Part model, mm, in its own coordinate system. A direction names the side the tool comes from. Coordinates: 2 decimals unless noted, no trailing zeros. Loops run counter-clockwise (first coordinate to the right, second up) from the corner with the lowest first, then second, coordinate; pieces in that order, holes last. Notation, with made-up numbers: (63, -18) -> (67, -18) arc R32 cw to (67, 19) -> close; hole circle Ø6 at (-16, 37). An arc over 180 degrees is marked (long way). Use one line per item in the form item = value. Start each with the question number.
(1) 3-axis set-ups, long thin cutter, end or side, ignore diameter. For faces 1 (the flat face through (50.8, 13, 2)), 2 (the cylindrical face through (40.561, 37.325, 1.565)): which of +Z, -Z, +X, -X, +Y, -Y reach the whole face in a straight line?
(2) Band-saw the part on C-C on y = 19. Give the cut face in (x, z) (3 decimals).
(3) Drill centre lines: L1, parallel to Y at x = 12.7, z = 1.55; L2, parallel to X at y = 17.5, z = 2.65; L3, parallel to Y at x = 30, z = 1.85. Where is each one in solid material? Low to high. Write a range as [from, to].
(4) Band-saw the part on B-B on x = 12.7. Give the cut face in (y, z) (3 decimals), then the cut area to 3 significant figures.
(5) Mould opens along X. For faces 3 (the cylindrical face through (62, 36, 2)), 4 (the flat face through (13, 0, 2)), 5 (the flat face through (76.2, 25, 2)) say: +X half, -X half, draft (parallel to the pull), parting line (faces both ways), or undercut.
(6) Pin check, flat tips, straight feed: P1, Ø4.5, axis at x = 63.5, y = 38.1, coming from the -Z side; P2, Ø1, axis at x = 34, z = 1, coming from the -Y side. Stop position of each tip, or through.
(7) Band-saw the part on A-A on y = 12.7. Give the cut face in (x, z) (3 decimals).
(8) Band-saw the part on D-D on z = 1.35. Give the cut face in (x, y), then the cut area to 3 significant figures.
Autodesk Inventor part; units mm, degrees
ref_plane "YZ Plane" through (0, 0, 0) normal (1, 0, 0) x (0, 1, 0)
ref_plane "XZ Plane" through (0, 0, 0) normal (0, 1, 0) x (-1, 0, 0)
ref_plane "XY Plane" through (0, 0, 0) normal (0, 0, 1) x (1, 0, 0)
sketch "Sketch1" plane through (0, 0, 0) normal (0, 0, 1) x (1, 0, 0)
  line L0 (0, 0) -> (25.4, 0)
  line L1 (25.4, 0) -> (25.4, 25.4)
  line L2 (25.4, 50.8) -> (0, 50.8)
  line L3 (0, 50.8) -> (0, 0)
  line L4 (0, 25.4) -> (0, 50.8)
  line L5 (12.7, 0) -> (12.7, 12.7) construction
  line L6 (12.7, 12.7) -> (12.7, 38.1) construction
  line L7 (12.7, 38.1) -> (38.1, 38.1) construction
  circle A0 centre (12.7, 12.7) radius 2.5797
  circle A1 centre (12.7, 38.1) radius 2.5797
  circle A2 centre (38.1, 38.1) radius 2.5797
  line L8 (25.4, 25.4) -> (50.8, 25.4)
  line L9 (50.8, 25.4) -> (50.8, 0)
  line L10 (50.8, 0) -> (76.2, 0)
  line L11 (76.2, 0) -> (76.2, 50.8)
  line L12 (76.2, 50.8) -> (25.4, 50.8)
  line L13 (38.1, 38.1) -> (63.5, 38.1) construction
  line L14 (63.5, 38.1) -> (63.5, 12.7) construction
  circle A3 centre (63.5, 38.1) radius 2.5797
  circle A4 centre (63.5, 12.7) radius 2.5797
  dimension "d0" = 25.4
  dimension "d1" = 50.8
  dimension "d5" = 12.7
  dimension "d6" = 25.4
  dimension "d7" = 25.4
  dimension "d11" = 5.1594
  dimension "d14" = 25.4
  dimension "d15" = 25.4
  dimension "d16" = 25.4
  dimension "d17" = 25.4
extrude "Extrusion2" add sketch "Sketch1" along normal blind 3.175
properties part number "C-Bracket"
A:
q1.face_1 = +Z, -Z, -Y
q1.face_2 = +Z, -Z
q2.outline = (0, 0) -> (25.4, 0) -> (25.4, 3.175) -> (0, 3.175) -> close; (50.8, 0) -> (76.2, 0) -> (76.2, 3.175) -> (50.8, 3.175) -> close
q3.L1 = [0, 10.12], [15.28, 35.52], [40.68, 50.8]
q3.L2 = [0, 25.4], [50.8, 76.2]
q3.L3 = [25.4, 50.8]
q4.outline = (0, 0) -> (10.12, 0) -> (10.12, 3.175) -> (0, 3.175) -> close; (15.28, 0) -> (35.52, 0) -> (35.52, 3.175) -> (15.28, 3.175) -> close; (40.68, 0) -> (50.8, 0) -> (50.8, 3.175) -> (40.68, 3.175) -> close
q4.area = 129 mm²
q5.face_3 = undercut
q5.face_4 = draft
q5.face_5 = +X half
q6.P1 = through
q6.P2 = 25.4
q7.outline = (0, 0) -> (10.12, 0) -> (10.12, 3.175) -> (0, 3.175) -> close; (15.28, 0) -> (25.4, 0) -> (25.4, 3.175) -> (15.28, 3.175) -> close; (50.8, 0) -> (60.92, 0) -> (60.92, 3.175) -> (50.8, 3.175) -> close; (66.08, 0) -> (76.2, 0) -> (76.2, 3.175) -> (66.08, 3.175) -> close
q8.outline = (0, 0) -> (25.4, 0) -> (25.4, 25.4) -> (50.8, 25.4) -> (50.8, 0) -> (76.2, 0) -> (76.2, 50.8) -> (0, 50.8) -> close; hole circle Ø5.16 at (12.7, 12.7); hole circle Ø5.16 at (12.7, 38.1); hole circle Ø5.16 at (38.1, 38.1); hole circle Ø5.16 at (63.5, 12.7); hole circle Ø5.16 at (63.5, 38.1)
q8.area = 3,120 mm²
